Study the drawing (mm; zero at the part's minimum x, y, z) and answer. A direction names the side the tool comes from. Round coordinates to 2 decimals unless told otherwise and drop trailing zeros. Order: outer loops, then holes, each group sorted by start corner. A loop starts at its lowest first (then second) coordinate and runs counter-clockwise, first axis right, second up. Notation, with made-up numbers: (36.25, 44.5) - (67.25, 44.5) arc R24 cw to (67.25, 60.5) - close; hole circle Ø10 at (52, 12). An arc over 180 degrees is marked (long way). Put each result on its own line as item: value.
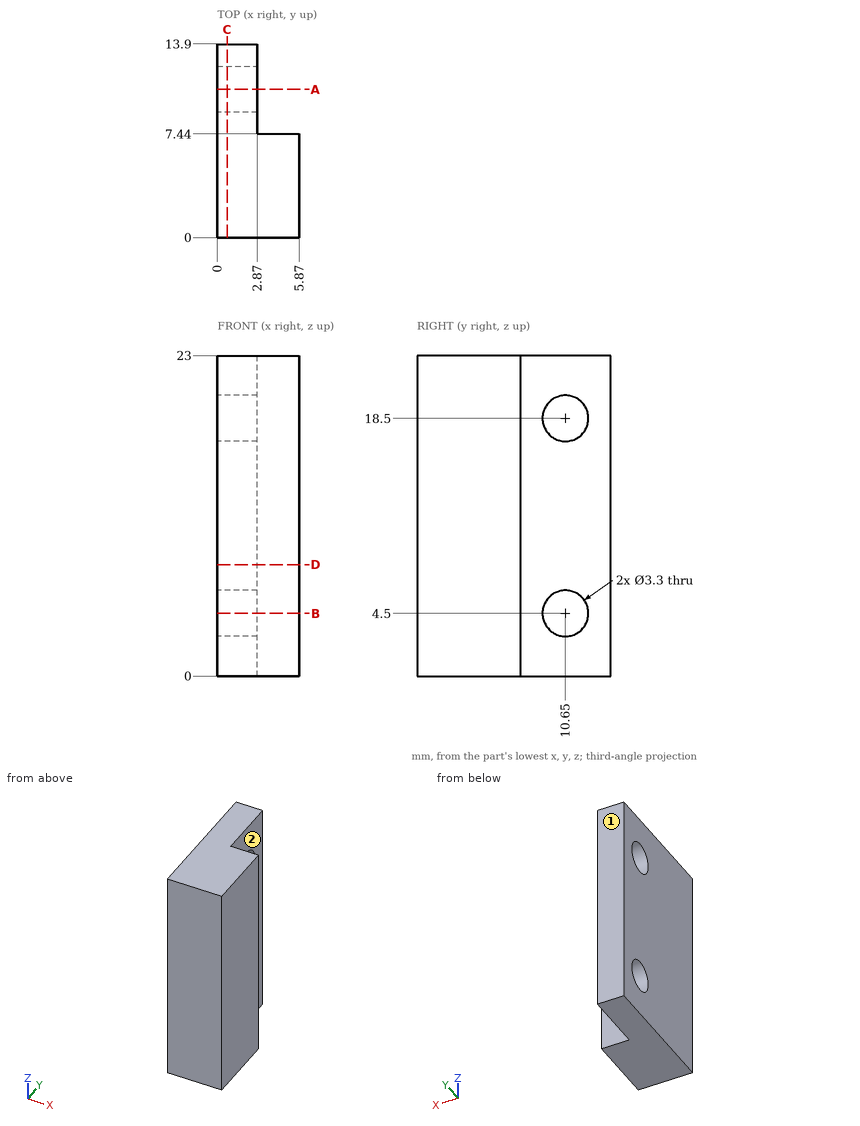
1) Given pin 1 Ø1.5 at (x, y) = (2.5, 3) entering from -Z; pin 2 Ø3 at (y, z) = (10, 7.5) entering from +X; pin 3 Ø2.5 at (y, z) = (10.65, 4.5) entering from -X, each flat-ended and moving along its own axis, determine where each tip first touches the part or whether it passes through.
Findings below:
pin 1: stops at z = 0
pin 2: stops at x = 2.87
pin 3: passes through
2) For the marked faces 1 and 2, determine the directions among +Z, -Z, +X, -X, +Y, -Y from which every point of the face is accessible in a straight line to the end or side of a thin tool.
Findings below:
face 1: +Z, -Z, +X, -X, +Y
face 2: +Z, -Z, +X, +Y
3) A cutting plane is placed at A-A on y = 10.65. Write down the section's boundary in (x, z).
Findings below:
outline: (0, 0) - (2.87, 0) - (2.87, 2.85) - (0, 2.85) - close; (0, 6.15) - (2.87, 6.15) - (2.87, 16.85) - (0, 16.85) - close; (0, 20.15) - (2.87, 20.15) - (2.87, 23) - (0, 23) - close
4) A cutting plane is placed at D-D on z = 8. Write down the section's boundary in (x, y).
Findings below:
outline: (0, 0) - (5.87, 0) - (5.87, 7.44) - (2.87, 7.44) - (2.87, 13.9) - (0, 13.9) - close
5) A cutting plane is placed at C-C on x = 0.7. Write down the section's boundary in (y, z).
Findings below:
outline: (0, 0) - (13.9, 0) - (13.9, 23) - (0, 23) - close; hole circle Ø3.3 at (10.65, 4.5); hole circle Ø3.3 at (10.65, 18.5)
6) Straight lines are drawn through the part: L1, parallel to Z at x = 1.15, y = 10.65; L2, parallel to Y at x = 3.3, z = 7.5; L3, parallel to Y at x = 2, z = 5. For each, find the intervals that lie inside material, in ascending order. Write a range as from..to.
Findings below:
L1: z = 0..2.85, 6.15..16.85, 20.15..23
L2: y = 0..7.44
L3: y = 0..9.08, 12.22..13.9
7) A cutting plane is placed at B-B on z = 4.5. Write down the section's boundary in (x, y).
Findings below:
outline: (0, 0) - (5.87, 0) - (5.87, 7.44) - (2.87, 7.44) - (2.87, 9) - (0, 9) - close; (0, 12.3) - (2.87, 12.3) - (2.87, 13.9) - (0, 13.9) - close
